Read the model definition and answer for the solid it produces. Units are mm, in the model's axes. A direction names the side the tool comes from. Round coordinates to 2 decimals unless told otherwise and drop trailing zeros. Order: outer loops, then holes, each group sorted by start corner. A loop starts at its lowest first (then second) coordinate and runs counter-clockwise, first axis right, second up. Notation, with made-up numbers: (-8, 31.25) - (39, 31.25) arc R27 ccw to (39, 63.25) - close; hole circle Ø5 at (-17.5, 84). An arc over 180 degrees is marked (long way). Put each result on its own line as item: value. Start each with the question number.
Q1. Find the intervals of material crossed by line 1 along X through (y, z) = (27, -36); line 2 along Z through (x, y) = (-28, 22); line 3 along Z through (x, y) = (34, 28.25), in increasing order. Write a range as from..to.
Q2. Which of the six approach directions +Z, -Z, +X, -X, +Y, -Y give full straight-line access (tool end or side, diameter ignored) to faces 4 (the face through (85.865, 15, 56)), 5 (the face through (-6, 15, -24.422)), 6 (the face through (88.865, 15, 1))?
Q3. Section C-C on x = -67.5 is taken. Give the vertices of the cut face in (y, z), then the cut area to 3 significant figures.
Q4. For a pull along X with two mould halves and no side action, classify faces 1 (the face through (-85.865, 15, 56)), 2 (the face through (-1, 30, -1)), 3 (the face through (-88.865, 15, 1)) as pulls with the +X half, pulls with the -X half, needs draft (parallel to the pull), parting line crosses it, or undercut.
Q5. Section A-A on x = -13.5 is taken. Give the vertices of the cut face in (y, z), then the cut area to 3 significant figures.
Q6. Section B-B on y = 19.5 is taken. Give the vertices of the cut face in (x, z).
Q7. Each of these flat-tipped pins is pushed along its axis until it touches: pin 1 Ø3 at (x, y) = (-46, 17) entering from +Z; pin 2 Ø11 at (x, z) = (-23, 55) entering from -Y. Where does it stop, or does it pass through?
from build123d import *

# Parameters (mm, degrees)
SKETCH1_W           = 177.730901972
SKETCH1_H           = 122.376165744
BOSS_EXTRUDE1_DEPTH = 30
SKETCH2_W           = 171.730901972
SKETCH2_H           = 24
CUT_EXTRUDE1_DEPTH  = 10
CUT_EXTRUDE2_DEPTH  = 112.986828978


with BuildPart() as part:
    # Sketch1 → Boss-Extrude1 (new body)
    with BuildSketch(Plane(origin=(0, 0, 0), x_dir=(1, 0, 0), z_dir=(0, 1, 0))):
        Rectangle(SKETCH1_W, SKETCH1_H)
    extrude(amount=BOSS_EXTRUDE1_DEPTH)

    # Sketch2 → Cut-Extrude1 (cut)
    with BuildSketch(Plane.XY.offset(61.188082872)):
        with Locations((0, 15)):
            Rectangle(SKETCH2_W, SKETCH2_H)
    extrude(amount=-CUT_EXTRUDE1_DEPTH, mode=Mode.SUBTRACT)

    # Sketch3 → Cut-Extrude2 (cut, through all)
    with BuildSketch(Plane(origin=(0, 30, 0), x_dir=(1, 0, 0), z_dir=(0, 1, 0))):
        with BuildLine():
            Line((-52.291434111, 46.257807098), (38.691830368, 46.257807098))
            ThreePointArc((38.691830368, 46.257807098), (49.609822105, 35.339815361), (38.691830368, 24.421823623))
            Line((38.691830368, 24.421823623), (-52.291434111, 24.421823623))
            ThreePointArc((-52.291434111, 24.421823623), (-63.209425848, 35.339815361), (-52.291434111, 46.257807098))
        make_face()
    extrude(amount=-CUT_EXTRUDE2_DEPTH, mode=Mode.SUBTRACT)


solid = part.part
Findings:
1. line 1: -88.87..-63.19, 49.59..88.87
1. line 2: -61.19..-46.26, -24.42..51.19
1. line 3: -61.19..-46.26, -24.42..61.19
2. face 4: +Z
2. face 5: +Y, -Y
2. face 6: +Z, -Z, +X, +Y, -Y
3. outline: (0, -61.19) - (30, -61.19) - (30, 61.19) - (27, 61.19) - (27, 51.19) - (3, 51.19) - (3, 61.19) - (0, 61.19) - close
3. area: 3,430 mm2
4. face 1: undercut
4. face 2: needs draft
4. face 3: pulls with the -X half
5. outline: (0, -61.19) - (30, -61.19) - (30, -46.26) - (0, -46.26) - close; (0, -24.42) - (30, -24.42) - (30, 61.19) - (27, 61.19) - (27, 51.19) - (3, 51.19) - (3, 61.19) - (0, 61.19) - close
5. area: 2,780 mm2
6. outline: (-88.87, -61.19) - (88.87, -61.19) - (88.87, 61.19) - (85.87, 61.19) - (85.87, 51.19) - (-85.87, 51.19) - (-85.87, 61.19) - (-88.87, 61.19) - close; hole (-52.29, -46.26) - (38.69, -46.26) arc R10.92 ccw to (38.69, -24.42) - (-52.29, -24.42) arc R10.92 ccw to start
7. pin 1: z = 51.19
7. pin 2: y = 0
